```python
from build123d import *
from build123d.topology import SkipClean

# Parameters (mm, degrees)
BOSS_EXTRU_1_DEPTH      = 5.8
ESQUISSE2_R             = 1.5
ESQUISSE2_R_2           = 6.4
ENL_V_MAT_EXTRU_1_DEPTH = 5.8
ESQUISSE3_W             = 42
ESQUISSE3_H             = 20.5
ENL_V_MAT_EXTRU_2_DEPTH = 5.8


with BuildPart() as part:
    # Esquisse1 → Boss.-Extru.1 (new body)
    with BuildSketch(Plane(origin=(0, 0, 0), x_dir=(1, 0, 0), z_dir=(0, 1, 0))):
        Polygon((0, 0), (-18.5, 0), (-18.5, -33), (-52, -56.345309326), (-52, -73.345309326), (-23, -92.941227268), (-4, -127), (0, -127), align=None)
    boss_extru_1 = extrude(amount=BOSS_EXTRU_1_DEPTH)

    # Esquisse2 → Enlèv. mat.-Extru.1 (cut)
    with BuildSketch(Plane(origin=(0, 5.8, 0), x_dir=(1, 0, 0), z_dir=(0, 1, 0))):
        with Locations(Location((-13.5, -5, 0), (0, 0, 270))):
            Circle(ESQUISSE2_R)
        with Locations((0, -19)):
            Circle(ESQUISSE2_R_2)
        with Locations(Location((-13.5, -32, 0), (0, 0, 270))):
            Circle(ESQUISSE2_R)
    enl_v_mat_extru_1 = extrude(amount=-ENL_V_MAT_EXTRU_1_DEPTH, mode=Mode.SUBTRACT)

    # Symétrie2: Boss.-Extru.1, Enlèv. mat.-Extru.1 across plane
    with SkipClean():  # the faces are left unmerged after this step: merging them gives an invalid solid
        add(boss_extru_1.mirror(Plane(origin=(0, 5.8, 0), x_dir=(0, 0, 1), z_dir=(-1, 0, 0))))
        add(enl_v_mat_extru_1.mirror(Plane(origin=(0, 5.8, 0), x_dir=(0, 0, 1), z_dir=(-1, 0, 0))), mode=Mode.SUBTRACT)

    # Esquisse3 → Enlèv. mat.-Extru.2 (cut)
    with SkipClean():  # the faces are left unmerged after this step: merging them gives an invalid solid
        with BuildSketch(Plane(origin=(0, 5.8, 0), x_dir=(1, 0, 0), z_dir=(0, 1, 0))):
            with Locations((-9, -55.25)):
                Rectangle(ESQUISSE3_W, ESQUISSE3_H)
        extrude(amount=-ENL_V_MAT_EXTRU_2_DEPTH, mode=Mode.SUBTRACT)


solid = part.part
```
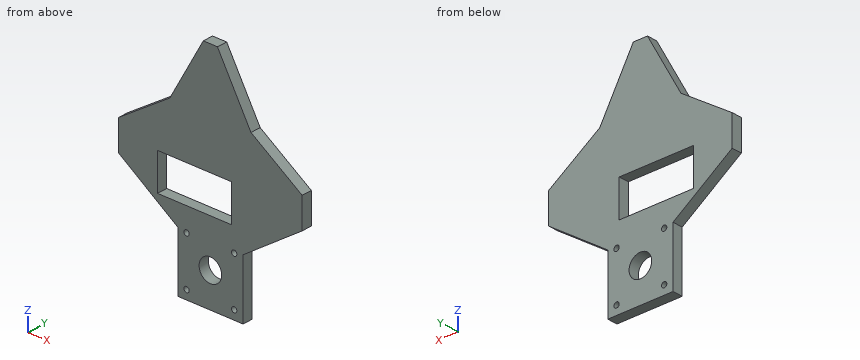
CAD build for the part. Positions are in the model's coordinates, mm. Round coordinates to 2 decimals unless told otherwise and drop trailing zeros. Write each loop counter-clockwise with the first axis right and the second up, starting at its lowest first coordinate (ties: lowest second). Pieces come first, ordered by that corner, then holes. Notation, with made-up numbers: (-6, -8.5) - (40, -8.5) arc R18 cw to (40, 5.5) - close; hole circle Ø1 at (38, 52). An arc over 180 degrees is marked (long way). Write item = value, one per line. Start each with the question number.
Q1. Band-saw the part on C-C (z = 5). Give the cut face in (x, y), then the cut area to 3 significant figures.
Q2. Drop flat-ended pins along their axis: pin 1 (2 mm diameter, centred on x = 29.5, y = 3, fed in from +Z); pin 2 (3 mm diameter, centred on x = -20.5, y = 2, fed in from -Z); pin 3 (1.7 mm diameter, centred on y = 3, z = 10.5, fed in from +X). Give the stop position or say it passes through.
Q3. Probe L1, parallel to X at y = 4.2, z = 32; L2, parallel to X at y = 5.2, z = 33; L3, parallel to Z at x = 13.5, y = 2.6. List the from-to ranges inside material, lowest first. Write a range as from..to.
Q4. Band-saw the part on A-A (z = 61.5). Give the cut face in (x, y).
Q5. Band-saw the part on B-B (y = 3.95). Give the cut face in (x, z), then the cut area to 3 significant figures.
Q6. Band-saw the part on D-D (x = 13.5). Give the cut face in (y, z).
Answers below:
q1.outline = (-18.5, 0) - (-15, 0) - (-15, 5.8) - (-18.5, 5.8) - close; (-12, 0) - (12, 0) - (12, 5.8) - (-12, 5.8) - close; (15, 0) - (18.5, 0) - (18.5, 5.8) - (15, 5.8) - close
q1.area = 180 mm2
q2.pin_1 = 89.22
q2.pin_2 = 33.35
q2.pin_3 = 18.5
q3.L1 = -18.5..-15, -12..12, 15..18.5
q3.L2 = -18.5..-14.62, -12.38..12.38, 14.62..18.5
q3.L3 = 0..3.5, 6.5..30.5, 33.5..109.97
q4.outline = (-52, 0) - (-30, 0) - (-30, 5.8) - (-52, 5.8) - close; (12, 0) - (52, 0) - (52, 5.8) - (12, 5.8) - close
q5.outline = (-52, 56.35) - (-18.5, 33) - (-18.5, 0) - (18.5, 0) - (18.5, 33) - (52, 56.35) - (52, 73.35) - (23, 92.94) - (4, 127) - (-4, 127) - (-23, 92.94) - (-52, 73.35) - close; hole (-30, 45) - (12, 45) - (12, 65.5) - (-30, 65.5) - close; hole circle Ø3 at (-13.5, 5); hole circle Ø3 at (-13.5, 32); hole circle Ø12.8 at (0, 19); hole circle Ø3 at (13.5, 5); hole circle Ø3 at (13.5, 32)
q5.area = 6,010 mm2
q6.outline = (0, 0) - (5.8, 0) - (5.8, 3.5) - (0, 3.5) - close; (0, 6.5) - (5.8, 6.5) - (5.8, 30.5) - (0, 30.5) - close; (0, 33.5) - (5.8, 33.5) - (5.8, 109.97) - (0, 109.97) - close
